Build history of the part. All positions in model axes, mm. A direction names the side the tool comes from. Coordinates: 2 decimals unless noted, no trailing zeros. Order: outer loops, then holes, each group sorted by start corner. A loop starts at its lowest first (then second) coordinate and runs counter-clockwise, first axis right, second up. Notation, with made-up numbers: (-14, -30.75) -> (2, -30.75) arc R7 ccw to (2, -19.75) -> close; hole circle Ø1 at (15, 15.25). An arc over 180 degrees is marked (long way). Write each question's results on one line, items separated by ' | '.
from build123d import *

# Parameters (mm, degrees)
BOSS_EXTRUDE1_DEPTH = 42
BOSS_EXTRUDE2_DEPTH = 46
SKETCH3_W           = 20
SKETCH3_H           = 10
BOSS_EXTRUDE3_DEPTH = 31
SKETCH4_W           = 10
SKETCH4_H           = 20
BOSS_EXTRUDE4_DEPTH = 21.387158
SKETCH6_R           = 2.5
CUT_EXTRUDE1_DEPTH  = 21


with BuildPart() as part:
    # Sketch1 → Boss-Extrude1 (new body)
    with BuildSketch(Plane.XY):
        Polygon((0, -4.144365492), (10, -4.144365492), (10, -35.531523796), (53, -35.531523796), (53, -2.113321439), (63, -2.113321439), (63, -25.531523796), (108, -25.531523796), (108, -35.531523796), (63, -35.531523796), (63, -45.531523796), (0, -45.531523796), (0, -35.531523796), (-45, -35.531523796), (-45, -25.531523796), (0, -25.531523796), align=None)
    extrude(amount=BOSS_EXTRUDE1_DEPTH)

    # Sketch2 → Boss-Extrude2 (add)
    with BuildSketch(Plane.XY.offset(42)):
        Polygon((-45, -25.531523796), (10, -25.531523796), (10, -35.531523796), (16, -35.531523796), (16, -45.531523796), (0, -45.531523796), (0, -35.531523796), (-45, -35.531523796), align=None)
        Polygon((53, -25.531523796), (108, -25.531523796), (108, -35.531523796), (63, -35.531523796), (63, -45.531523796), (47, -45.531523796), (47, -35.531523796), (53, -35.531523796), align=None)
    extrude(amount=BOSS_EXTRUDE2_DEPTH)

    # Sketch3 → Boss-Extrude3 (add)
    with BuildSketch(Plane.ZY.offset(-47)):
        with Locations((78, -40.531523796)):
            Rectangle(SKETCH3_W, SKETCH3_H)
    extrude(amount=BOSS_EXTRUDE3_DEPTH)

    # Sketch4 → Boss-Extrude4 (add)
    with BuildSketch(Plane(origin=(0, -25.531523796, 0), x_dir=(1, 0, 0), z_dir=(0, 1, 0))):
        with Locations((5, -78)):
            Rectangle(SKETCH4_W, SKETCH4_H)
        with Locations((58, -78)):
            Rectangle(SKETCH4_W, SKETCH4_H)
    extrude(amount=BOSS_EXTRUDE4_DEPTH)

    # Sketch6 → Cut-Extrude1 (cut, through all)
    with BuildSketch(Plane(origin=(0, -25.531523796, 0), x_dir=(1, 0, 0), z_dir=(0, 1, 0))):
        with Locations((-36.5, -54.5)):
            Circle(SKETCH6_R)
        with Locations((-8.5, -54.5)):
            Circle(SKETCH6_R)
        with Locations((-36.5, -33.5)):
            Circle(SKETCH6_R)
        with Locations((-8.5, -33.5)):
            Circle(SKETCH6_R)
    extrude(amount=-CUT_EXTRUDE1_DEPTH, mode=Mode.SUBTRACT)


solid = part.part
Item 1: Slice it at B-B, the plane x = -8.5. List the corners of the cut face in (y, z).
Answer:
outline: (-35.53, 0) -> (-25.53, 0) -> (-25.53, 31) -> (-35.53, 31) -> close; (-35.53, 36) -> (-25.53, 36) -> (-25.53, 52) -> (-35.53, 52) -> close; (-35.53, 57) -> (-25.53, 57) -> (-25.53, 88) -> (-35.53, 88) -> close
Item 2: Tool access for faces 4 (the flat face through (58, -15, 68)), 5 (the flat face through (0, -15, 78)), 6 (the flat face through (16, -40, 55)): list every direction of +Z, -Z, +X, -X, +Y, -Y with a clear straight run to the whole face (end or side of a thin tool).
Answer:
face 4: +X, -X, +Y | face 5: +Z, -Z, -X, +Y | face 6: +Y, -Y
Item 3: Drill centre lines: line 1 (X direction, y = -31.75, z = 54.5); line 2 (X direction, y = -6, z = 40); line 3 (X direction, y = -35.5, z = 13). Where is each one in solid material? Low to high. Write a range as from..to.
Answer:
line 1: x = -45..-39, -34..-11, -6..10, 53..108 | line 2: x = 0..10, 53..63 | line 3: x = -45..10, 53..108
Item 4: Slice it at D-D, the plane y = -7. List the corners of the cut face in (x, z).
Answer:
outline: (0, 0) -> (10, 0) -> (10, 42) -> (0, 42) -> close; (0, 68) -> (10, 68) -> (10, 88) -> (0, 88) -> close; (53, 0) -> (63, 0) -> (63, 42) -> (53, 42) -> close; (53, 68) -> (63, 68) -> (63, 88) -> (53, 88) -> close
Item 5: Slice it at C-C, the plane z = 54.5. List the corners of the cut face in (x, y).
Answer:
outline: (-45, -35.53) -> (-39, -35.53) -> (-39, -25.53) -> (-45, -25.53) -> close; (-34, -35.53) -> (-11, -35.53) -> (-11, -25.53) -> (-34, -25.53) -> close; (-6, -35.53) -> (0, -35.53) -> (0, -45.53) -> (16, -45.53) -> (16, -35.53) -> (10, -35.53) -> (10, -25.53) -> (-6, -25.53) -> close; (47, -45.53) -> (63, -45.53) -> (63, -35.53) -> (108, -35.53) -> (108, -25.53) -> (53, -25.53) -> (53, -35.53) -> (47, -35.53) -> close
Item 6: Pull direction Z, two halves, no side cores. Call faces 1 (the flat face through (31, -37, 88)), 2 (the cylindrical face through (-9.04, -30.46, 56.94)), 3 (the flat face through (63, -15, 78)): released by +Z, released by -Z, zero draft, split by the parting line, or undercut.
Answer:
face 1: released by +Z | face 2: undercut | face 3: zero draft
Item 7: Slice it at A-A, the plane y = -27. List the corners of the cut face in (x, z), and give its area (3 significant figures).
Answer:
outline: (-45, 0) -> (10, 0) -> (10, 88) -> (-45, 88) -> close; (53, 0) -> (108, 0) -> (108, 88) -> (53, 88) -> close; hole circle Ø5 at (-36.5, 33.5); hole circle Ø5 at (-36.5, 54.5); hole circle Ø5 at (-8.5, 33.5); hole circle Ø5 at (-8.5, 54.5) | area: 9,600 mm^2
Item 8: Pin check, flat tips, straight feed: pin 1 (8 mm diameter, centred on x = 19, z = 35, fed in from +Y); pin 2 (6 mm diameter, centred on y = -16, z = 74.5, fed in from +X); pin 3 (16.5 mm diameter, centred on y = -15, z = 24, fed in from -X). Stop position of each tip, or through.
Answer:
pin 1: stops at y = -35.53 | pin 2: stops at x = 63 | pin 3: stops at x = 0
